Here's how the part is built. I have some questions about the finished solid (model axes, mm). A direction names the side the tool comes from. Give positions to 0.01 mm unless a question says otherwise; leave off trailing zeros. Loops run counter-clockwise (first coordinate to the right, second up) from the corner with the lowest first, then second, coordinate; pieces in that order, holes last.
Q1. Suppose I cut it at B-B (z = -6.5). List the corners of the cut face in (x, y) for me, and give its area (3 significant figures).
Q2. Suppose I cut it at C-C (z = -12). List the corners of the cut face in (x, y) for me, and give its area (3 significant figures).
Q3. Suppose I cut it at D-D (y = 30). List the corners of the cut face in (x, z) for me.
Q4. Suppose I cut it at A-A (x = 32). List the corners of the cut face in (y, z) for me.
Q5. I need wall thicknesses on probe 1 along Z at (x, y) = (-3, 19); probe 2 along Y at (x, z) = (3.5, -1); probe 3 along X at (y, z) = (26, -3.5). Which ranges of each line are inside material? Lowest first, please.
Q6. I'm going to push flat-ended pins straight in: P1, Ø8, axis at x = 9.5, y = 26.5, coming from the +Z side; P2, Ø6.5, axis at y = 5, z = -4.5, coming from the +X side; P3, Ø4, axis at y = 6.5, z = -9, coming from the -X side; P4, Ø4, axis at x = 31.5, z = -5, coming from the +Y side. Where does each tip first touch, or does it pass through?
Q7. Thinking about a two-plate mould opening in Z: for faces 1 (the face through (14, 14, 0)), 2 (the face through (-0.8, 18.6, -6.6)), 3 (the face through (-1, 20.08, -6.43)), which applies, pulls with the +Z half, pulls with the -Z half, needs draft (parallel to the pull), parting line crosses it, or undercut?
Q8. For faces 4 (the face through (0, 9, -6)), 5 (the face through (0, 25, -6)), 6 (the face through (29.8, 18.6, -6.6)), 7 (the face through (29.8, 21.6, -6.6)), which set-ups out of +Z, -Z, +X, -X, +Y, -Y let a thin tool reach every point of the face, with its end or its side?
```python
from build123d import *

# Parameters (mm, degrees)
SKETCH_1_W      = 29
SKETCH_1_H      = 13
EXTRUDE_2_DEPTH = 29.2
EXTRUDE_3_DEPTH = 3
SKETCH_3_R      = 2.5
EXTRUDE_4_DEPTH = 3.6


with BuildPart() as part:
    # 草图1 → 凸台-拉伸2 (new body)
    with BuildSketch(Plane(origin=(0, 0, 0), x_dir=(1, 0, 0), z_dir=(0, 1, 0))):
        with Locations((14.5, 6.5)):
            Rectangle(SKETCH_1_W, SKETCH_1_H)
    extrude(amount=EXTRUDE_2_DEPTH)

    # 草图2 → 凸台-拉伸3 (add)
    with BuildSketch(Plane(origin=(0, 18.6, 0), x_dir=(-1, 0, 0), z_dir=(0, -1, 0))):
        with BuildLine():
            Line((-29, 0), (-29, 13))
            Line((-29, 13), (-33.706494839, 13))
            Line((-33.706494839, 13), (-33.706494839, 7.543012639))
            ThreePointArc((-33.706494839, 7.543012639), (-30, 6.5), (-33.706494839, 5.456987361))
            Line((-33.706494839, 5.456987361), (-33.706494839, 0))
            Line((-33.706494839, 0), (-29, 0))
        make_face()
        with BuildLine():
            Line((4.706494839, 13), (0, 13))
            Line((0, 13), (0, 0))
            Line((0, 0), (4.706494839, 0))
            Line((4.706494839, 0), (4.706494839, 5.456987361))
            ThreePointArc((4.706494839, 5.456987361), (1, 6.5), (4.706494839, 7.543012639))
            Line((4.706494839, 7.543012639), (4.706494839, 13))
        make_face()
    extrude(amount=-EXTRUDE_3_DEPTH)

    # 草图3 → 凸台-拉伸4 (add)
    with BuildSketch(Plane(origin=(0, 29.2, 0), x_dir=(1, 0, 0), z_dir=(0, 1, 0))):
        with Locations(Location((6.5, 6.5, 0), (0, 0, 90))):
            Circle(SKETCH_3_R)
    extrude(amount=EXTRUDE_4_DEPTH)


solid = part.part
```
Solutions:
1. outline: (-1, 18.6) - (0, 18.6) - (0, 0) - (29, 0) - (29, 18.6) - (30, 18.6) - (30, 21.6) - (29, 21.6) - (29, 29.2) - (9, 29.2) - (9, 32.8) - (4, 32.8) - (4, 29.2) - (0, 29.2) - (0, 21.6) - (-1, 21.6) - close
1. area: 871 mm2
2. outline: (-4.71, 18.6) - (0, 18.6) - (0, 0) - (29, 0) - (29, 18.6) - (33.71, 18.6) - (33.71, 21.6) - (29, 21.6) - (29, 29.2) - (0, 29.2) - (0, 21.6) - (-4.71, 21.6) - close
2. area: 875 mm2
3. outline: circle Ø5 at (6.5, -6.5)
4. outline: (18.6, -13) - (21.6, -13) - (21.6, -8.5) - (18.6, -8.5) - close; (18.6, -4.5) - (21.6, -4.5) - (21.6, 0) - (18.6, 0) - close
5. probe 1: z = -13 to -8.5, -4.5 to 0
5. probe 2: y = 0 to 29.2
5. probe 3: x = 0 to 29
6. P1: stops at z = 0
6. P2: stops at x = 29
6. P3: stops at x = 0
6. P4: stops at y = 21.6
7. face 1: pulls with the +Z half
7. face 2: needs draft
7. face 3: undercut
8. face 4: +Z, -Z, -X, -Y
8. face 5: +Z, -Z, -X, +Y
8. face 6: +Z, -Z, +X, -Y
8. face 7: +Z, -Z, +X, +Y
